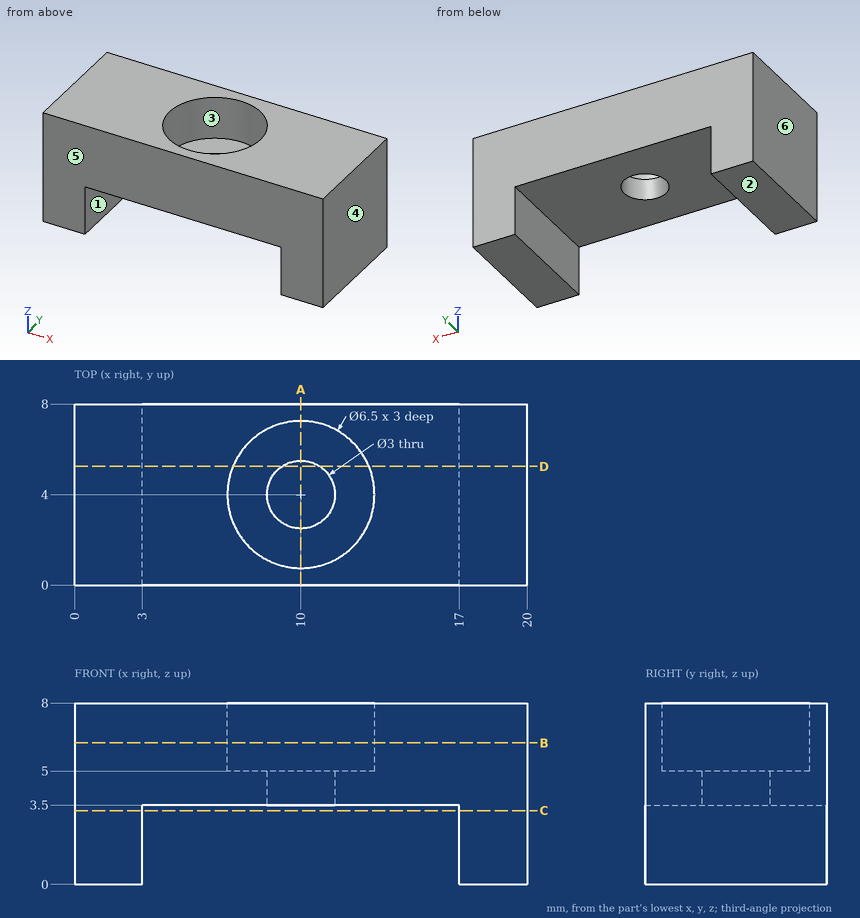
Source: three-view drawing plus pictorial views. Frame: mm from the lowest corner of the part. A direction names the side the tool comes from. Give positions to 0.01 mm unless a question says otherwise; leave off trailing zeros. Order: outer loops, then holes, each group sorted by start corner. A loop starts at its lowest first (then second) coordinate and runs counter-clockwise, first axis right, second up. Notation, with made-up numbers: (-17, 19.25) -> (10, 19.25) arc R24 cw to (10, 46.25) -> close; hole circle Ø11 at (38, -0.5). An arc over 180 degrees is marked (long way). Put each result on its own line as item: value.
Q1. Material intervals for L1, parallel to Y at x = 10, z = 4.25; L2, parallel to X at y = 3.75, z = 2.25; L3, parallel to Z at x = 16, y = 2, sorted ascending.
Here are the results:
L1: y = 0 to 2.5, 5.5 to 8
L2: x = 0 to 3, 17 to 20
L3: z = 3.5 to 8
Q2. Section D-D, the plane y = 5.25. Return loops of the section in (x, z), then the cut area to 3 significant figures.
Here are the results:
outline: (0, 0) -> (3, 0) -> (3, 3.5) -> (9.17, 3.5) -> (9.17, 5) -> (7, 5) -> (7, 8) -> (0, 8) -> close; (10.83, 3.5) -> (17, 3.5) -> (17, 0) -> (20, 0) -> (20, 8) -> (13, 8) -> (13, 5) -> (10.83, 5) -> close
area: 90.5 mm^2
Q3. Section A-A, the plane x = 10. Return loops of the section in (y, z), then the cut area to 3 significant figures.
Here are the results:
outline: (0, 3.5) -> (2.5, 3.5) -> (2.5, 5) -> (0.75, 5) -> (0.75, 8) -> (0, 8) -> close; (5.5, 3.5) -> (8, 3.5) -> (8, 8) -> (7.25, 8) -> (7.25, 5) -> (5.5, 5) -> close
area: 12.0 mm^2
Q4. Pin query (flat end, axial travel): pin 1 (4 mm diameter, centred on x = 10, y = 4, fed in from -Z); pin 2 (4 mm diameter, centred on y = 4.5, z = 1.5, fed in from -X); pin 3 (1.5 mm diameter, centred on x = 11.5, y = 3.5, fed in from +Z). Return the tip coordinate at first contact, or that it passes through.
Here are the results:
pin 1: stops at z = 3.5
pin 2: stops at x = 0
pin 3: stops at z = 5
Q5. Section C-C, the plane z = 3.25. Return loops of the section in (x, y), then the cut area to 3 significant figures.
Here are the results:
outline: (0, 0) -> (3, 0) -> (3, 8) -> (0, 8) -> close; (17, 0) -> (20, 0) -> (20, 8) -> (17, 8) -> close
area: 48.0 mm^2
Q6. Section B-B, the plane z = 6.25. Return loops of the section in (x, y).
Here are the results:
outline: (0, 0) -> (20, 0) -> (20, 8) -> (0, 8) -> close; hole circle Ø6.5 at (10, 4)
Q7. Draft query along X for the marked faces 3, 4, 5 and 6. Return one class per face: released by +X, released by -X, zero draft, split by the parting line, or undercut.
Here are the results:
face 3: undercut
face 4: released by +X
face 5: zero draft
face 6: released by -X
Q8. Reachability of the marked faces 1 and 2 from +Z, -Z, +X, -X, +Y, -Y: full face, straight path, thin tool, end or side. Return the list, or none.
Here are the results:
face 1: -Z, +Y, -Y
face 2: -Z, +X, -X, +Y, -Y
